```python
from build123d import *

# Parameters (mm, degrees)
SKETCH1_R                = 16
BOSS_EXTRUDE1_DEPTH      = 10
CUT_EXTRUDE1_DEPTH       = 10
BOSS_EXTRUDE2_DEPTH      = 10
FILLET1_R                = 0.5
CIRPATTERN1_COUNT        = 19
CIRPATTERN1_ANGLE        = 350
FILLET1_OF_CIRPATTERN1_R = 0.5
SKETCH4_R                = 2
CUT_EXTRUDE2_DEPTH       = 11
SKETCH5_R                = 1.2
CUT_EXTRUDE3_DEPTH       = 11


with BuildPart() as part:
    # Sketch1 → Boss-Extrude1 (new body)
    with BuildSketch(Plane(origin=(0, 0, 0), x_dir=(1, 0, 0), z_dir=(0, 1, 0))):
        with BuildLine():
            Line((162.614680299, 55.320508076), (165.373914051, 35.511756749))
            Line((165.373914051, 35.511756749), (159.055986536, 8))
            ThreePointArc((159.055986536, 8), (172.912392996, 16), (186.768799457, 8))
            Line((186.768799457, 8), (186.768799457, 38))
            Line((186.768799457, 38), (176.768799457, 55.320508076))
            Line((176.768799457, 55.320508076), (165.373914051, 88.413658222))
            Line((165.373914051, 88.413658222), (156.912392996, 93.743072959))
            ThreePointArc((156.912392996, 93.743072959), (152.296156749, 93.493334083), (150.998552799, 89.056191919))
            Line((150.998552799, 89.056191919), (162.614680299, 55.320508076))
        make_face()
        with Locations((172.912392996, 0)):
            Circle(SKETCH1_R)
    extrude(amount=BOSS_EXTRUDE1_DEPTH)

    # Sketch2 → Cut-Extrude1 (cut)
    with BuildSketch(Plane(origin=(0, 10, 0), x_dir=(1, 0, 0), z_dir=(0, 1, 0))):
        with BuildLine():
            Line((150.998552799, 89.056191919), (152.951961726, 83.383080466))
            ThreePointArc((152.951961726, 83.383080466), (154.811812989, 87.196340656), (150.998552799, 89.056191919))
        make_face()
        with BuildLine():
            Line((153.928666189, 80.546524739), (155.882075116, 74.873413285))
            ThreePointArc((155.882075116, 74.873413285), (157.741926379, 78.686673476), (153.928666189, 80.546524739))
        make_face()
        with BuildLine():
            Line((156.858779579, 72.036857559), (158.812188506, 66.363746105))
            ThreePointArc((158.812188506, 66.363746105), (160.672039769, 70.177006295), (156.858779579, 72.036857559))
        make_face()
        with BuildLine():
            Line((159.788892969, 63.527190378), (161.742301896, 57.854078925))
            ThreePointArc((161.742301896, 57.854078925), (163.602153159, 61.667339115), (159.788892969, 63.527190378))
        make_face()
        with BuildLine():
            Line((162.659719683, 54.997166876), (163.487489808, 49.054541478))
            ThreePointArc((163.487489808, 49.054541478), (166.044917445, 52.43973924), (162.659719683, 54.997166876))
        make_face()
        with BuildLine():
            Line((163.901374871, 46.083228779), (165.373914051, 35.511756749))
            Line((165.373914051, 35.511756749), (169.018329151, 38.934948035))
            ThreePointArc((169.018329151, 38.934948035), (169.935727078, 41.535482158), (168.342564959, 43.786311148))
            Line((168.342564959, 43.786311148), (163.901374871, 46.083228779))
        make_face()
        with BuildLine():
            Line((168.037228767, 28.862370748), (164.702457837, 32.587864386))
            Line((164.702457837, 32.587864386), (162.314311904, 22.18855388))
            Line((162.314311904, 22.18855388), (166.940336365, 24.085893514))
            ThreePointArc((166.940336365, 24.085893514), (168.725824948, 26.190051977), (168.037228767, 28.862370748))
        make_face()
        with BuildLine():
            Line((164.977626621, 15.539167879), (161.642855691, 19.264661516))
            Line((161.642855691, 19.264661516), (159.254709758, 8.86535101))
            Line((159.254709758, 8.86535101), (163.880734219, 10.762690644))
            ThreePointArc((163.880734219, 10.762690644), (165.666222802, 12.866849107), (164.977626621, 15.539167879))
        make_face()
    extrude(amount=-CUT_EXTRUDE1_DEPTH, mode=Mode.SUBTRACT)

    # Sketch3 → Boss-Extrude2 (add)
    with BuildSketch(Plane(origin=(0, 10, 0), x_dir=(1, 0, 0), z_dir=(0, 1, 0))):
        with BuildLine():
            Line((190.096751538, 1.503436562), (188.851508166, 1.394491884))
            ThreePointArc((188.851508166, 1.394491884), (188.912392996, 0), (188.851508166, -1.394491884))
            Line((188.851508166, -1.394491884), (190.096751538, -1.503436562))
            ThreePointArc((190.096751538, -1.503436562), (191.072085254, -1.370072078), (191.894309206, -0.82876836))
            ThreePointArc((191.894309206, -0.82876836), (191.912392996, 0), (191.894309206, 0.82876836))
            ThreePointArc((191.894309206, 0.82876836), (191.072085254, 1.370072078), (190.096751538, 1.503436562))
        make_face()
    boss_extrude2 = extrude(amount=-BOSS_EXTRUDE2_DEPTH)

    # Fillet1
    fillet1_edges = [part.edges().sort_by_distance(p)[0] for p in [
        (188.851508166, 5, 1.394491884),
        (188.851508166, 5, -1.394491884),
    ]]
    fillet(fillet1_edges, radius=FILLET1_R)

    # CirPattern1: Boss-Extrude2 ×19 about axis, 8 skipped
    cirpattern1_axis = Axis((172.912392996, 0, 0), (0, -1, 0))
    add([boss_extrude2.rotate(cirpattern1_axis, i * CIRPATTERN1_ANGLE / (CIRPATTERN1_COUNT - 1)) for i in range(1, CIRPATTERN1_COUNT) if i not in (11, 12, 13, 14, 15, 16, 17, 18)])

    # Fillet1 of CirPattern1
    fillet1_of_cirpattern1_edges = [part.edges().sort_by_distance(p)[0] for p in [
        (187.478200052, 5, 6.620971592),
        (188.406632365, 5, 3.991058305),
        (184.443362059, 5, 11.092193312),
        (186.194319884, 5, 8.921346207),
        (180.093179879, 5, 14.298122245),
        (182.466930463, 5, 12.833971084),
        (174.923881264, 5, 15.873056257),
        (177.649649531, 5, 15.282617594),
        (169.52513104, 5, 15.637341732),
        (172.291987056, 5, 15.98796724),
        (164.512767711, 5, 13.617866759),
        (167.005094639, 5, 14.869560388),
        (160.458554405, 5, 10.044993995),
        (162.392051099, 5, 12.054974341),
        (157.824957537, 5, 5.326283064),
        (158.979068931, 5, 7.865270529),
        (156.912392996, 5, 0),
        (157.155468948, 5, 2.778370843),
        (157.824957537, 5, -5.326283064),
        (157.129270235, 5, -2.625459183),
    ]]
    fillet(fillet1_of_cirpattern1_edges, radius=FILLET1_OF_CIRPATTERN1_R)

    # Sketch4 → Cut-Extrude2 (cut, through all)
    with BuildSketch(Plane(origin=(0, 10, 0), x_dir=(1, 0, 0), z_dir=(0, 1, 0))):
        with Locations((172.912392996, 0)):
            Circle(SKETCH4_R)
    extrude(amount=-CUT_EXTRUDE2_DEPTH, mode=Mode.SUBTRACT)

    # Sketch5 → Cut-Extrude3 (cut, through all)
    with BuildSketch(Plane(origin=(0, 10, 0), x_dir=(1, 0, 0), z_dir=(0, 1, 0))):
        with Locations((169.092781716, 61.667339115)):
            Circle(SKETCH5_R)
        with Locations((177.33165748, 41.535482158)):
            Circle(SKETCH5_R)
        with Locations((175.039520306, 17.401914698)):
            Circle(SKETCH5_R)
        with Locations((159.593070103, 87.196340656)):
            Circle(SKETCH5_R)
    extrude(amount=-CUT_EXTRUDE3_DEPTH, mode=Mode.SUBTRACT)


solid = part.part
```
Geometry: final body of the model. Coordinates: model frame, mm. A direction names the side the tool comes from. Round coordinates to 2 decimals unless told otherwise and drop trailing zeros. Loops run counter-clockwise (first coordinate to the right, second up) from the corner with the lowest first, then second, coordinate; pieces in that order, holes last.
Item 1: Section A-A, the plane y = 9. State how many separate pieces and enclosed holes the cut face has, plus the area to 3 significant figures.
Checked values:
separate pieces: 1
enclosed holes: 5
area: 2,090 mm2
Item 2: Section B-B, the plane z = -52. Output: boundary loops of the cut face in (x, y).
Checked values:
outline: (166.07, 0) - (178.69, 0) - (178.69, 10) - (166.07, 10) - close
Item 3: Contact query for flat-ended pins moving along their axis: P1, Ø1.5, axis at y = 2.5, z = -77, coming from the -X side; P2, Ø3, axis at x = 159.59, z = -87.2, coming from the -Y side; P3, Ø1, axis at x = 184, y = 3.5, coming from the +Z side; P4, Ø0.8, axis at x = 156, y = 7.5, coming from the -Z side. Output: stop coordinate, or through.
Checked values:
P1: stops at x = 157.53
P2: stops at y = 0
P3: stops at z = 15.78
P4: stops at z = -94.27
Item 4: Mould query, pull axis Z, two halves, no side actions, for faces 1 (the cylindrical face through (152.351, 4.93, -93.536)), 2 (the cylindrical face through (186.17, 5.07, 12.46)), 3 (the flat face through (163.69, 4.93, -47.59)). Classes: released by +Z, released by -Z, zero draft, split by the parting line, or undercut.
Checked values:
face 1: split by the parting line
face 2: released by +Z
face 3: undercut
Item 5: Line query: L1, parallel to Z at x = 164, y = 3; L2, parallel to Z at x = 187, y = 5.75; L3, parallel to Z at x = 189, y = 5.5. Output: solid intervals per line, ascending.
Checked values:
L1: z = -89.28 to -54.88, -49.17 to -46.03, -22.88 to -16.63, -10.81 to 13.29, 14.45 to 16.78
L2: z = -7.59 to 7.59, 9.46 to 12.58
L3: z = -1.53 to 1.53, 4.14 to 7.27
Item 6: Reachability of faces 4 (the flat face through (186.769, 5, -23)), 5 (the flat face through (161.535, 5.07, -9.801)), 6 (the cylindrical face through (160.693, 5.07, -70.114)) from +Z, -Z, +X, -X, +Y, -Y: full face, straight path, thin tool, end or side. Return the list, or none.
Checked values:
face 4: -Z, +X, +Y, -Y
face 5: -X, +Y, -Y
face 6: +Y, -Y
